Geometry: final body of the model. Coordinates: model frame, mm. Face numbers are marked on the shaded views. Round coordinates to 2 decimals unless told otherwise and drop trailing zeros. Loops run counter-clockwise (first coordinate to the right, second up) from the corner with the lowest first, then second, coordinate; pieces in that order, holes last. Notation, with made-up numbers: (26.5, 63.5) - (39.5, 63.5) arc R21 ccw to (39.5, 100.5) - close; hole circle Ø11 at (17, 71). An arc over 180 degrees is marked (long way). Answer as a JSON object with one key per item and string values. Group by question number.
Item 1: Section B-B (z = -28). Return the cut outline in (x, y), plus the area to 3 significant figures.
Item 2: Section D-D (x = -6.5). Return the cut outline in (y, z), plus the area to 3 significant figures.
Item 3: First-contact query: pin 1 (3 mm diameter, centred on y = -5.5, z = -34.5, fed in from +X); pin 2 (1.5 mm diameter, centred on y = 9.5, z = -38, fed in from +X); pin 3 (10 mm diameter, centred on y = -5.5, z = -51.5, fed in from +X). Flat tips, straight axial feed; report the tip coordinate or a pass-through.
Item 4: Section A-A (x = 0). Return the cut outline in (y, z).
Item 5: Line query: line 1 (Z direction, x = -3, y = 12); line 2 (X direction, y = -0.5, z = -49); line 3 (X direction, y = 3, z = 2). Output: solid intervals per line, ascending.
Item 6: Draft query along X for the marked faces 1, 2 and 3. Return one class per face: released by +X, released by -X, zero draft, split by the parting line, or undercut.
Item 7: Section C-C (y = 6). Return the cut outline in (x, z).
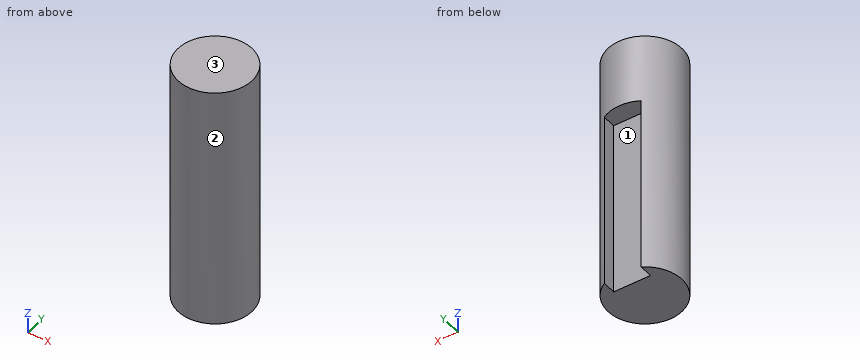
```python
from build123d import *

# Parameters (mm, degrees)
SKETCH1_W          = 15
SKETCH1_H          = 100
CUT_EXTRUDE1_DEPTH = 72


with BuildPart() as part:
    # Sketch1 → Revolve1 (revolve)
    with BuildSketch(Plane(origin=(0, 0, 0), x_dir=(1, 0, 0), z_dir=(0, 1, 0))):
        with Locations((7.5, 22)):
            Rectangle(SKETCH1_W, SKETCH1_H)
    revolve(axis=Axis((0, 0, -72), (0, 0, 1)))

    # Sketch2 → Cut-Extrude1 (cut)
    with BuildSketch(Plane(origin=(0, 0, -72), x_dir=(-1, 0, 0), z_dir=(0, 0, -1))):
        with BuildLine():
            Line((-7.5, 12.990381057), (-7.5, 7.5))
            Line((-7.5, 7.5), (7.5, 7.5))
            Line((7.5, 7.5), (7.5, 12.990381057))
            ThreePointArc((7.5, 12.990381057), (0, 15), (-7.5, 12.990381057))
        make_face()
    extrude(amount=-CUT_EXTRUDE1_DEPTH, mode=Mode.SUBTRACT)


solid = part.part
```
Values:
{
 "1": {"outline": "(-7.5, 7.5) - (-7.5, 12.99) arc R15 ccw (long way) to (7.5, 12.99) - (7.5, 7.5) - close", "area": "604 mm^2"},
 "2": {"outline": "(-13.52, -72) - (7.5, -72) - (7.5, 0) - (13.52, 0) - (13.52, 28) - (-13.52, 28) - close", "area": "2,270 mm^2"},
 "3": {"pin 1": "stops at x = 14.46", "pin 2": "stops at x = 12.18", "pin 3": "stops at x = 14.99"},
 "4": {"outline": "(-15, -72) - (7.5, -72) - (7.5, 0) - (15, 0) - (15, 28) - (-15, 28) - close"},
 "5": {"line 1": "z = 0 to 28", "line 2": "x = -14.99 to 14.99", "line 3": "x = -14.7 to 14.7"},
 "6": {"face 1": "undercut", "face 2": "split by the parting line", "face 3": "zero draft"},
 "7": {"outline": "(-13.75, -72) - (13.75, -72) - (13.75, 28) - (-13.75, 28) - close"}
}
